Can you work these out from the model? Positions are in its coordinate system, mm. Coordinates: 2 decimals unless noted, no trailing zeros. Write each loop counter-clockwise with the first axis right and the second up, starting at its lowest first coordinate (ties: lowest second). Pieces come first, ordered by that corner, then holes. Notation, with made-up numbers: (-23.5, 48.25) - (29.5, 48.25) arc R19 cw to (29.5, 77.25) - close; hole circle Ø9 at (42.5, 87). An arc over 180 degrees is marked (long way). Write each question's results on one line, items separated by ' | '. Start each with the question number.
```python
from build123d import *

# Parameters (mm, degrees)
F0_R     = 14
F1_DEPTH = 12
F1_TAPER = 1
F2_R     = 16
F3_DEPTH = 16
F4_R     = 4.5
F5_DEPTH = 5


with BuildPart() as f1:
    # F0 (on Top) → F1 (new body)
    with BuildSketch(Plane.XY):
        Circle(F0_R)
    extrude(amount=F1_DEPTH, taper=F1_TAPER)

    # F2 (on Front) → F3 (cut, symmetric)
    with BuildSketch(Plane.XZ):
        with Locations((0, 19)):
            Circle(F2_R)
    extrude(amount=F3_DEPTH, both=True, mode=Mode.SUBTRACT)

    # F4 (on face) → F5 (cut)
    with BuildSketch(Plane(origin=(0, 0, 0), x_dir=(1, 0, 0), z_dir=(0, 0, -1))):
        Circle(F4_R)
    extrude(amount=-F5_DEPTH, mode=Mode.SUBTRACT)


solid = f1.part
```
Q1. I'm going to push flat-ended pins straight in: pin 1 Ø1 at (y, z) = (-7.5, 6) entering from -X; pin 2 Ø3 at (y, z) = (10, 1.5) entering from -X; pin 3 Ø5 at (y, z) = (-10.5, 1) entering from -X. Where does each tip first touch, or does it pass through?
Q2. If we section it at A-A (z = 6.75): Please give me the cut outline in (x, y), then the cut area to 3 significant figures.
Q3. Thinking about a two-plate mould opening in X: for faces 1 (the face through (3.442, -3.295, 3.375)), 2 (the face through (-3.3, 3.3, 0)), 3 (the face through (6.44, -12.37, 3.11)), 4 (the face through (2.08, 3.99, 1.81)), which applies, pulls with the +X half, pulls with the -X half, needs draft (parallel to the pull), parting line crosses it, or undercut?
Q4. I need wall thicknesses on line 1 along Y through (x, z) = (0, 2.95); line 2 along X through (y, z) = (-1.5, 2.5); line 3 along Y through (x, z) = (0, 1.75). Which ranges of each line are inside material? Lowest first, please. Write a range as from..to.
Q5. If we section it at B-B (z = 1.75): Please give me the cut outline in (x, y), then the cut area to 3 significant figures.
Answer list:
1) pin 1: stops at x = -12 | pin 2: stops at x = -11.09 | pin 3: stops at x = -11.47
2) outline: (-10.29, -9.32) - (-10.29, 9.32) arc R13.88 ccw to start; (10.29, -9.32) arc R13.88 ccw to (10.29, 9.32) - close | area: 91.8 mm2
3) face 1: undercut | face 2: needs draft | face 3: parting line crosses it | face 4: undercut
4) line 1: y = -13.95..-4.5, 4.5..13.95 | line 2: x = -13.88..-4.24, 4.24..13.88 | line 3: y = -13.97..-4.5, 4.5..13.97
5) outline: circle Ø27.94 at (0, 0); hole circle Ø9 at (0, 0) | area: 549 mm2
